Geometry: final body of the model. Coordinates: model frame, mm. Coordinates: 2 decimals unless noted, no trailing zeros. Order: outer loops, then holes, each group sorted by start corner. A loop starts at its lowest first (then second) coordinate and runs counter-clockwise, first axis right, second up. Notation, with made-up numbers: M 67.5,45.25 L 87.5,45.25 A19 ccw 87.5,65.25 Z; hole C 50.25,29 d8. An arc over 180 degrees is marked long. Use CSV: the item, a comma, the result in double quotes. Start each with the question number.
1. Section query A-A on x = -9. Return the cut outline in (y, z).
2. Section query B-B on y = 25. Return the cut outline in (x, z), and give its area (3 significant figures).
3. Material intervals for line 1 (Y direction, x = -8, z = 0.75); line 2 (X direction, y = -29, z = 0.55), sorted ascending.
4. Section query C-C on z = 0.8. State how many separate pieces and enclosed holes the cut face has, and give its area (3 significant figures).
5. First-contact query: P1, Ø3, axis at x = 63, y = 9.5, coming from the -Z side. Flat tip, straight axial feed; report the tip coordinate or a pass-through.
from build123d import *

# Parameters (mm, degrees)
F0_W     = 170
F0_H     = 130
F1_DEPTH = 3


with BuildPart() as f1:
    # F0 (on Top) → F1 (new body)
    with BuildSketch(Plane.XY):
        Rectangle(F0_W, F0_H)
        with BuildLine():
            ThreePointArc((-81, -19.5), (-81.353553, -18.646447), (-80.5, -19))
            Line((-80.5, -19), (-78.3, -19))
            ThreePointArc((-78.3, -19), (-77.8, -18.5), (-77.3, -19))
            ThreePointArc((-77.3, -19), (-77.446447, -19.353553), (-77.8, -19.5))
            Line((-77.8, -19.5), (-77.8, -30.5))
            ThreePointArc((-77.8, -30.5), (-77.446447, -30.646447), (-77.3, -31))
            ThreePointArc((-77.3, -31), (-77.8, -31.5), (-78.3, -31))
            Line((-78.3, -31), (-80.5, -31))
            ThreePointArc((-80.5, -31), (-81.353553, -31.353553), (-81, -30.5))
            Line((-81, -30.5), (-81, -19.5))
        make_face(mode=Mode.SUBTRACT)
        with BuildLine():
            ThreePointArc((-25, -58.3), (-25.353553, -57.446447), (-24.5, -57.8))
            Line((-24.5, -57.8), (24.5, -57.8))
            ThreePointArc((24.5, -57.8), (25, -57.3), (25.5, -57.8))
            ThreePointArc((25.5, -57.8), (25.353553, -58.153553), (25, -58.3))
            Line((25, -58.3), (25, -60.5))
            ThreePointArc((25, -60.5), (25.353553, -60.646447), (25.5, -61))
            ThreePointArc((25.5, -61), (25, -61.5), (24.5, -61))
            Line((24.5, -61), (-24.5, -61))
            ThreePointArc((-24.5, -61), (-25.353553, -61.353553), (-25, -60.5))
            Line((-25, -60.5), (-25, -58.3))
        make_face(mode=Mode.SUBTRACT)
        with BuildLine():
            ThreePointArc((77.8, -19.5), (77.446447, -18.646447), (78.3, -19))
            Line((78.3, -19), (80.5, -19))
            ThreePointArc((80.5, -19), (81, -18.5), (81.5, -19))
            ThreePointArc((81.5, -19), (81.353553, -19.353553), (81, -19.5))
            Line((81, -19.5), (81, -30.5))
            ThreePointArc((81, -30.5), (81.353553, -30.646447), (81.5, -31))
            ThreePointArc((81.5, -31), (81, -31.5), (80.5, -31))
            Line((80.5, -31), (78.3, -31))
            ThreePointArc((78.3, -31), (77.446447, -31.353553), (77.8, -30.5))
            Line((77.8, -30.5), (77.8, -19.5))
        make_face(mode=Mode.SUBTRACT)
        with BuildLine():
            ThreePointArc((-80.5, 19), (-81.353553, 18.646447), (-81, 19.5))
            Line((-81, 19.5), (-81, 30.5))
            ThreePointArc((-81, 30.5), (-81.353553, 31.353553), (-80.5, 31))
            Line((-80.5, 31), (-78.3, 31))
            ThreePointArc((-78.3, 31), (-77.8, 31.5), (-77.3, 31))
            ThreePointArc((-77.3, 31), (-77.446447, 30.646447), (-77.8, 30.5))
            Line((-77.8, 30.5), (-77.8, 19.5))
            ThreePointArc((-77.8, 19.5), (-77.446447, 19.353553), (-77.3, 19))
            ThreePointArc((-77.3, 19), (-77.8, 18.5), (-78.3, 19))
            Line((-78.3, 19), (-80.5, 19))
        make_face(mode=Mode.SUBTRACT)
        with BuildLine():
            ThreePointArc((77.8, 30.5), (77.446447, 31.353553), (78.3, 31))
            Line((78.3, 31), (80.5, 31))
            ThreePointArc((80.5, 31), (81, 31.5), (81.5, 31))
            ThreePointArc((81.5, 31), (81.353553, 30.646447), (81, 30.5))
            Line((81, 30.5), (81, 19.5))
            ThreePointArc((81, 19.5), (81.353553, 19.353553), (81.5, 19))
            ThreePointArc((81.5, 19), (81, 18.5), (80.5, 19))
            Line((80.5, 19), (78.3, 19))
            ThreePointArc((78.3, 19), (77.446447, 18.646447), (77.8, 19.5))
            Line((77.8, 19.5), (77.8, 30.5))
        make_face(mode=Mode.SUBTRACT)
        with BuildLine():
            ThreePointArc((-25, 60.5), (-25.353553, 61.353553), (-24.5, 61))
            Line((-24.5, 61), (24.5, 61))
            ThreePointArc((24.5, 61), (25, 61.5), (25.5, 61))
            ThreePointArc((25.5, 61), (25.353553, 60.646447), (25, 60.5))
            Line((25, 60.5), (25, 58.3))
            ThreePointArc((25, 58.3), (25.353553, 58.153553), (25.5, 57.8))
            ThreePointArc((25.5, 57.8), (25, 57.3), (24.5, 57.8))
            Line((24.5, 57.8), (-24.5, 57.8))
            ThreePointArc((-24.5, 57.8), (-25.353553, 57.446447), (-25, 58.3))
            Line((-25, 58.3), (-25, 60.5))
        make_face(mode=Mode.SUBTRACT)
    extrude(amount=F1_DEPTH)


solid = f1.part
Results list:
1,outline,"M -65,0 L -61,0 L -61,3 L -65,3 Z; M -57.8,0 L 57.8,0 L 57.8,3 L -57.8,3 Z; M 61,0 L 65,0 L 65,3 L 61,3 Z"
2,outline,"M -85,0 L -81,0 L -81,3 L -85,3 Z; M -77.8,0 L 77.8,0 L 77.8,3 L -77.8,3 Z; M 81,0 L 85,0 L 85,3 L 81,3 Z"
2,area,"491 mm²"
3,line 1,"y = -65 to -61, -57.8 to 57.8, 61 to 65"
3,line 2,"x = -85 to -81, -77.8 to 77.8, 81 to 85"
4,separate pieces,"1"
4,enclosed holes,"6"
4,area,"21,600 mm²"
5,P1,"stops at z = 0"
